The model under review builds one solid part; all positions refer to its coordinate system, in mm. A direction names the side the tool comes from. Give positions to 0.01 mm unless a question says otherwise; leave off trailing zeros. Loops run counter-clockwise (first coordinate to the right, second up) from the corner with the lowest first, then second, coordinate; pieces in that order, holes last. Notation, with made-up numbers: M -6,68.5 L 3,68.5 A17 ccw 3,90.5 Z; hole C 79.5,-30.75 d7. An arc over 180 degrees is marked long. One line per item, written item: value. Start each with the question number.
Q1. For faces 1 (the face through (76.65, 8, 119)), 2 (the face through (76, 8, 3.537)), 3 (the face through (84.906, 8, 8)), 4 (the face through (75.36, 8.26, 119.95)), 5 (the face through (64, 8, 123.27)), list the 3-axis set-ups (+Z, -Z, +X, -X, +Y, -Y) from which the entire face can be reached by the end or side of a thin tool; tool diameter is ignored.
Q2. We need section D-D on x = 134. Write out the cut boundary in (y, z) (3 decimals), plus the area to 3 significant figures.
Q3. Mouldability with a two-part tool opening along X and no side actions: class faces 6 (the face through (55.22, 8.26, 120.93)), 7 (the face through (64, 36.83, 38)), 8 (the face through (68.79, 18.16, 54.91)) as released by +X, released by -X, zero draft, split by the parting line, or undercut.
Q4. We need section B-B on z = 38.1. Write out the cut boundary in (x, y) (3 decimals).
Q5. We need section A-A on y = 13. Give the number of separate pieces and of enclosed holes in the cut face, plus the area to 3 significant figures.
Q6. For pin 1 (1 mm diameter, centred on x = 112, z = 88.5, fed in from +Y); pin 2 (2.5 mm diameter, centred on x = 79.5, z = 6.5, fed in from +Y); pin 3 (13.5 mm diameter, centred on x = 77.5, y = 11.5, fed in from +Z); pin 4 (4 mm diameter, centred on x = 125.73, z = 120.65, fed in from -Y) (3 decimals), all flat-tipped, find the tip position at first contact; note any pin that passes through.
Q7. We need section C-C on y = 26. Write out the cut boundary in (x, z).
Q8. To check wall thickness, follow line 1 along X through (y, z) = (5, 119); line 2 along Y through (x, z) = (131.5, 89.5) (3 decimals); line 3 along X through (y, z) = (17, 81). State the ranges of each line that lie inside material, in increasing order. Write a range as from..to.
```python
from build123d import *

# Parameters (mm, degrees)
SKETCH1_W      = 251.46
SKETCH1_H      = 127
SKETCH1_R      = 1.4605
SKETCH1_R_2    = 1.5875
EXTRUDE1_DEPTH = 1.905
SKETCH2_R      = 17.62125
EXTRUDE2_DEPTH = 36.83
SKETCH3_W      = 25.4
SKETCH3_H      = 9.398
SKETCH3_R      = 2.54
SKETCH3_W_2    = 17.018
SKETCH3_H_2    = 8.0717042
EXTRUDE3_DEPTH = 16.764


with BuildPart() as part:
    # Sketch1 → Extrude1 (new body)
    with BuildSketch(Plane(origin=(0, 0, 0), x_dir=(1, 0, 0), z_dir=(0, 1, 0))):
        with Locations((125.73, -63.5)):
            Rectangle(SKETCH1_W, SKETCH1_H)
        with Locations(Location((28.575, -120.65, 0), (0, 0, 270))):
            Circle(SKETCH1_R, mode=Mode.SUBTRACT)
        with Locations(Location((28.575, -6.35, 0), (0, 0, 270))):
            Circle(SKETCH1_R, mode=Mode.SUBTRACT)
        with Locations(Location((245.11, -6.35, 0), (0, 0, 270))):
            Circle(SKETCH1_R, mode=Mode.SUBTRACT)
        with Locations(Location((245.11, -120.65, 0), (0, 0, 270))):
            Circle(SKETCH1_R, mode=Mode.SUBTRACT)
        with Locations(Location((125.73, -6.35, 0), (0, 0, 270))):
            Circle(SKETCH1_R, mode=Mode.SUBTRACT)
        with Locations(Location((125.73, -120.65, 0), (0, 0, 270))):
            Circle(SKETCH1_R, mode=Mode.SUBTRACT)
        with Locations(Location((18.415, -44.45, 0), (0, 0, 270))):
            Circle(SKETCH1_R_2, mode=Mode.SUBTRACT)
        with Locations(Location((18.415, -79.755956549, 0), (0, 0, 270))):
            Circle(SKETCH1_R_2, mode=Mode.SUBTRACT)
        with Locations(Location((18.415, -64.034066138, 0), (0, 0, 270))):
            Circle(SKETCH1_R_2, mode=Mode.SUBTRACT)
        with Locations(Location((18.415, -97.79, 0), (0, 0, 270))):
            Circle(SKETCH1_R_2, mode=Mode.SUBTRACT)
    extrude(amount=-EXTRUDE1_DEPTH)

    # Sketch2 → Extrude2 (add)
    with BuildSketch(Plane(origin=(0, 0, 0), x_dir=(1, 0, 0), z_dir=(0, 1, 0))):
        with Locations(Location((63.5, -76.2, 0), (0, 0, 270))):
            Circle(SKETCH2_R)
        with Locations(Location((63.5, -38.1, 0), (0, 0, 270))):
            Circle(SKETCH2_R)
    extrude(amount=EXTRUDE2_DEPTH)

    # Sketch3 → Extrude3 (add)
    # profile 1 of 2: a face of its own
    with BuildSketch(Plane(origin=(0, 0, 0), x_dir=(1, 0, 0), z_dir=(0, 1, 0))):
        with Locations((63.950056038, -118.57149124)):
            Rectangle(SKETCH3_W, SKETCH3_H)
        with Locations(Location((56.195547634, -118.584869875, 0), (0, 0, 270))):
            Circle(SKETCH3_R, mode=Mode.SUBTRACT)
        with Locations(Location((64.741474732, -118.584869875, 0), (0, 0, 270))):
            Circle(SKETCH3_R, mode=Mode.SUBTRACT)
        with Locations(Location((73.219619493, -118.584869875, 0), (0, 0, 270))):
            Circle(SKETCH3_R, mode=Mode.SUBTRACT)
    # profile 2 of 2: a face of its own
    with BuildSketch(Plane(origin=(0, 0, 0), x_dir=(1, 0, 0), z_dir=(0, 1, 0))):
        with Locations((76.396506794, -7.572762817)):
            Rectangle(SKETCH3_W_2, SKETCH3_H_2)
        with Locations(Location((71.865279643, -7.572762817, 0), (0, 0, 270))):
            Circle(SKETCH3_R, mode=Mode.SUBTRACT)
        with Locations(Location((80.836132406, -7.572762817, 0), (0, 0, 270))):
            Circle(SKETCH3_R, mode=Mode.SUBTRACT)
    extrude(amount=EXTRUDE3_DEPTH)


solid = part.part
```
Solved:
1. face 1: +Z, +X, +Y
1. face 2: -Z, +X, -X, +Y
1. face 3: +Z, -Z, +X, +Y
1. face 4: +Y
1. face 5: +Z, +X, -X, +Y
2. outline: M -1.905,0 L 0,0 L 0,127 L -1.905,127 Z
2. area: 242 mm2
3. face 6: undercut
3. face 7: zero draft
3. face 8: split by the parting line
4. outline: M 0,-1.905 L 251.46,-1.905 L 251.46,0 L 81.121,0 L 81.121,36.83 L 45.879,36.83 L 45.879,0 L 0,0 Z
5. separate pieces: 4
5. enclosed holes: 5
5. area: 2,230 mm2
6. pin 1: y = 0
6. pin 2: y = 16.76
6. pin 3: z = 123.27
6. pin 4: y = -1.905
7. outline: C 63.5,38.1 d35.24; C 63.5,76.2 d35.24
8. line 1: 51.25..53.69, 58.7..62.24, 67.25..70.71, 75.73..76.65
8. line 2: -1.905..0
8. line 3: 46.55..80.45
